The model under review builds one solid part; all positions refer to its coordinate system, in mm. Face numbers are marked on the shaded views. A direction names the side the tool comes from. Round coordinates to 2 decimals unless told otherwise and drop trailing zeros. Order: outer loops, then holes, each group sorted by start corner. A loop starts at its lowest first (then second) coordinate and runs counter-clockwise, first axis right, second up.
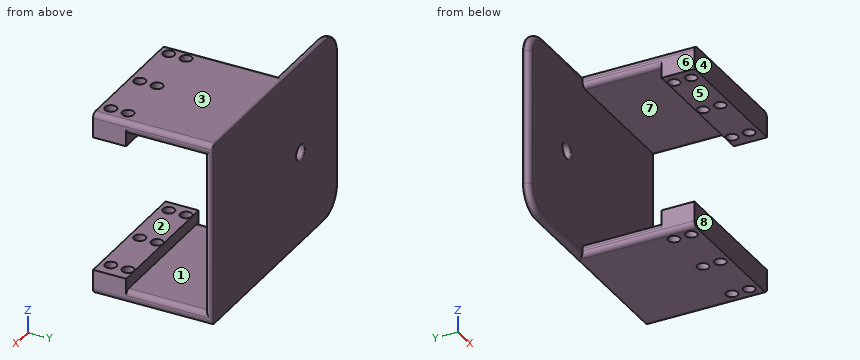
Autodesk Inventor part; units mm, degrees
ref_plane "Work Plane2" through (-91.43, -48.7723, -27.5) normal (0, 0, 1) x (1, 0, 0)
ref_plane "YZ Plane" through (0, 0, 0) normal (1, 0, 0) x (0, 1, 0)
ref_plane "XZ Plane" through (0, 0, 0) normal (0, 1, 0) x (-1, 0, 0)
ref_plane "Work Plane1" through (0, 0, -55) normal (0, 0, -1) x (1, 0, 0)
sketch "Sketch2" plane through (0, 0, -55) normal (0, 0, -1) x (1, 0, 0)
  circle A0 centre (23, 9) radius 2.35
  circle A1 centre (1, 9) radius 2.35
  circle A2 centre (-21, 9) radius 2.35
  circle A3 centre (-21, 16) radius 2.35
  circle A4 centre (1, 16) radius 2.35
  circle A5 centre (23, 16) radius 2.35
  circle A6 centre (-66, 12.5) radius 1.6
  circle A7 centre (63, 29.65) radius 1.6
  arc A8 (58.9857, 35) -> (49.7248, 32.4349) centre (58.9857, 17) ccw
  line L0 (33.2752, 22.5651) -> (49.7248, 32.4349)
  arc A9 (24.0143, 20) -> (33.2752, 22.5651) centre (24.0143, 38) ccw
  line L1 (-71, 20) -> (24.0143, 20)
  arc A10 (-71, 20) -> (-81, 10) centre (-71, 10) ccw
  line L2 (-81, 6.5495) -> (-81, 10)
  line L3 (-80.0877, 6.5495) -> (-81, 6.5495)
  line L4 (81, 6.5495) -> (-80.0877, 6.5495)
  line L5 (81, 20) -> (81, 6.5495)
  arc A11 (81, 20) -> (66, 35) centre (66, 20) ccw
  line L6 (58.9857, 35) -> (66, 35)
  line L7 (-21, 16) -> (-26, 16)
  line L8 (-21, 16) -> (-16, 16) construction
  line L9 (-26, 16) -> (-26, 20)
  line L10 (-26, 20) -> (29, 20)
  line L11 (29, 20) -> (29, 6.5495)
  line L12 (29, 6.5495) -> (-26, 6.5495)
  line L13 (-26, 6.5495) -> (-26, 20)
  point P0 (0, 0)
  dimension "d0" = 5
  dimension "d1" = 180
  dimension "d2" = 55
extrude "Extrusion1" add sketch "Sketch2" along normal blind 10 contours L10 L11 L4 L13 L9 L1
sketch "Sketch3" plane through (-26, -6.5495, -55) normal (0, 1, 0) x (1, 0, 0)
  line L0 (0, 0) -> (0, 10)
  line L1 (0, 10) -> (55, 10)
  line L2 (55, 10) -> (55, 5)
  line L3 (55, 5) -> (0, 5)
  line L4 (0, 5) -> (0, 10)
  point P0 (26, -55)
  dimension "d5" = 55
  dimension "d6" = 5
extrude "Extrusion2" add sketch "Sketch3" along normal blind 35
sketch "Sketch4" plane through (-26, -6.5495, -60) normal (0, 0, 1) x (1, 0, 0)
  line L0 (0, -13.4505) -> (0, 35)
  line L1 (0, 35) -> (55, 35)
  line L2 (55, 35) -> (55, 32)
  line L3 (55, 32) -> (0, 32)
  line L4 (0, 32) -> (0, 35)
  point P0 (26, 6.5495)
  dimension "d9" = 55
  dimension "d10" = 3
ref_plane "Work Plane2" through (-91.43, -48.7723, -27.5) normal (0, 0, 1) x (1, 0, 0)
extrude "Extrusion3" add sketch "Sketch4" along normal up to surface (32.5 mm away)
ref_plane "Work Plane3" through (-26, -6.5495, -27.5) normal (0, 0, 1) x (1, 0, 0)
mirror "Mirror1" about plane through (-26, -6.5495, -27.5) normal (0, 0, 1) of "Extrusion3", "Extrusion2", "Extrusion1"
ref_plane "Work Plane4" through (-26, 25.4505, -55) normal (0, 1, 0) x (1, 0, 0)
sketch "Sketch5" plane through (-26, 25.4505, -55) normal (0, 1, 0) x (1, 0, 0)
  line L0 (55, 5) -> (55, -60)
  line L1 (55, -27.5) -> (55, -65)
  line L2 (55, -27.5) -> (92.5, -27.5) construction
  line L3 (55, -65) -> (-40, -65)
  line L4 (-40, -65) -> (-40, 10)
  line L5 (-40, 10) -> (55, 10)
  line L6 (55, 10) -> (55, -65)
  line L7 (55, -65) -> (0, -65)
  line L8 (55, 10) -> (0, 10)
  line L9 (0, 10) -> (0, -65)
  line L10 (-12, 10) -> (-12, -65) construction
  line L11 (-48.9083, -27.5) -> (104.1186, -27.5) construction
  circle A0 centre (-12, -27.5) radius 3
  point P0 (26, -55)
  dimension "d16" = 90
  dimension "d21" = 0
  dimension "d22" = 0
  dimension "d23" = 40
  dimension "d24" = 28
  dimension "d25" = 6
extrude "Extrusion4" add sketch "Sketch5" along normal blind 3 contours L0 L1 L3 L9 L5 L6 | L9 L3 L4 L5 | A0
sketch "Sketch6" plane through (-26, 28.4505, -55) normal (0, 1, 0) x (1, 0, 0)
  point P0 (26, -55)
sketch "Sketch7" plane through (-26, 25.4505, -55) normal (0, 1, 0) x (1, 0, 0)
  point P0 (26, -55)
sketch "Sketch8" plane through (-26, 28.4505, -55) normal (0, 1, 0) x (1, 0, 0)
  line L0 (55, 10) -> (-40, 10)
  line L1 (-40, -65) -> (55, -65)
  line L2 (-12, 10) -> (-12, -65) construction
  line L3 (-40, 10) -> (-40, -65) construction
  line L4 (-40, -27.5) -> (55, -27.5) construction
  line L5 (55, 5) -> (55, -60) construction
  circle A0 centre (-12, -27.5) radius 3
  point P0 (26, -55)
  dimension "d26" = 6
extrude "Extrusion5" cut sketch "Sketch8" against normal blind 3 from surface at 0
fillet "Fillet1" radius 0.5 1 edges at (-41, 28.4505, -27.5)
fillet "Fillet2" radius 0.5 1 edges at (-41, 25.4505, -27.5)
fillet "Fillet3" radius 10 2 edges at (-66, 26.9505, 10) (-66, 26.9505, -65)
fillet "Fillet4" radius 2 12 edges at (-26, 9.4505, 5) (-26, 2.7253, 10) (29, 9.4505, 5) (29, 9.4505, -60) (-26, 2.7253, -65) (-26, 9.4505, -60) (-63.0711, 25.4505, -62.0711) (-66, 25.4505, -27.5) (-63.0711, 25.4505, 7.0711) (-41, 25.4505, 10) (-41, 25.4505, -65) (29, 25.4505, -27.5)
fillet "Fillet5" radius 2 2 edges at (29, 4.2253, -65) (29, 4.2253, 10)
fillet "Fillet6" radius 0.5 8 edges at (-63.0711, 28.4505, -62.0711) (-66, 28.4505, -27.5) (-63.0711, 28.4505, 7.0711) (-14.5, 28.4505, 10) (28.4142, 28.4505, 9.4142) (29, 28.4505, -27.5) (28.4142, 28.4505, -64.4142) (-14.5, 28.4505, -65)
properties part number "apriltag_head"
(1) Tool access review of the marked faces 5, 6, 7 and 8: name each direction out of +Z, -Z, +X, -X, +Y, -Y from which nothing blocks a thin tool from reaching the whole face with its end or side.
(2) We need section B-B (z = -27.5). Give the boundary of the cut face in (x, y), and give its area (3 significant figures).
(3) We need section A-A (y = 11). Give the boundary of the cut face in (x, z).
(4) Clearance check with flat-ended pins moving along their axes: P1, Ø12, axis at y = -6.5, z = 2, coming from the -X side; P2, Ø4, axis at x = 23, y = -16, coming from the +Z side; P3, Ø5.5, axis at x = 1, y = -9, coming from the +Z side; P4, Ø3, axis at x = 8, z = -41.5, coming from the -Y side. State where each tip first meets the part, or that it passes through.
(5) To check wall thickness, follow L1, parallel to X at y = -16, z = -62; L2, parallel to Y at x = -21, z = -62.5; L3, parallel to Z at x = -3, y = 22. State the ranges of each line that lie inside material, in increasing order.
(6) We need section C-C (x = -21). Count the separate pieces of the cut face and the enclosed holes in it, and give its area (3 significant figures).
(7) The part is to be moulded in two halves that separate along Z. For the marked faces 1, 2, 3 and 4, say which applies: pulls with the +Z half, pulls with the -Z half, needs draft (parallel to the pull), parting line crosses it, or undercut.
Verdict:
1. face 5: +X, -X, -Y
1. face 6: +Z, -Z, -X, -Y
1. face 7: +X, -X
1. face 8: +Z, -Z, +X, -X, -Y
2. outline: (-66, 27.45) arc R2 ccw to (-64, 25.45) - (-41.5, 25.45) arc R0.5 ccw to (-41, 25.95) - (-41, 27.95) arc R0.5 ccw to (-41.5, 28.45) - (-65.5, 28.45) arc R0.5 ccw to (-66, 27.95) - close; (-35, 25.95) arc R0.5 ccw to (-34.5, 25.45) - (27, 25.45) arc R2 ccw to (29, 27.45) - (29, 27.95) arc R0.5 ccw to (28.5, 28.45) - (-34.5, 28.45) arc R0.5 ccw to (-35, 27.95) - close
2. area: 265 mm2
3. outline: (-26, -63) arc R2 ccw to (-24, -65) - (27, -65) arc R2 ccw to (29, -63) - (29, -62) arc R2 ccw to (27, -60) - (-24, -60) arc R2 ccw to (-26, -62) - close; (-26, 7) arc R2 ccw to (-24, 5) - (27, 5) arc R2 ccw to (29, 7) - (29, 8) arc R2 ccw to (27, 10) - (-24, 10) arc R2 ccw to (-26, 8) - close
4. P1: stops at x = -26
4. P2: passes through
4. P3: stops at z = 10
4. P4: stops at y = 25.45
5. L1: x = -26 to -23.35, -18.65 to -1.35, 3.35 to 20.65, 25.35 to 29
5. L2: y = -20 to -18.35, -13.65 to -11.35, -6.65 to 28.45
5. L3: z = -65 to -60, 5 to 10
6. separate pieces: 5
6. enclosed holes: 0
6. area: 626 mm2
7. face 1: undercut
7. face 2: undercut
7. face 3: pulls with the +Z half
7. face 4: needs draft
